Autodesk Inventor part; units mm, degrees
ref_plane "YZ Plane" through (0, 0, 0) normal (1, 0, 0) x (0, 1, 0)
ref_plane "XZ Plane" through (0, 0, 0) normal (0, 1, 0) x (-1, 0, 0)
ref_plane "XY Plane" through (0, 0, 0) normal (0, 0, 1) x (1, 0, 0)
sketch "Sketch1" plane through (0, 0, 0) normal (0, 1, 0) x (-1, 0, 0)
  line L0 (0, 0) -> (355.6, 0)
  line L1 (355.6, 0) -> (355.6, -406.4)
  line L2 (355.6, -406.4) -> (0, -406.4)
  line L3 (0, -406.4) -> (0, 0)
  dimension "d0" = 355.6
  dimension "d1" = 406.4
extrude "Extrusion1" add sketch "Sketch1" along normal blind 152.4
sketch "Sketch2" plane through (0, 152.4, 0) normal (0, 1, 0) x (1, 0, 0)
  line L0 (-355.6, 0) -> (0, 0)
  line L1 (0, 0) -> (0, 406.4)
  line L2 (0, 406.4) -> (-355.6, 406.4)
  line L3 (-355.6, 406.4) -> (-355.6, 0)
  line L4 (-1.5875, 1.5875) -> (-354.0125, 1.5875)
  line L5 (-354.0125, 1.5875) -> (-354.0125, 404.8125)
  line L6 (-354.0125, 404.8125) -> (-1.5875, 404.8125)
  line L7 (-1.5875, 404.8125) -> (-1.5875, 1.5875)
  dimension "d4" = 1.5875
  dimension "d5" = 1.5875
  dimension "d6" = 1.5875
  dimension "d7" = 1.5875
extrude "Extrusion2" cut sketch "Sketch2" against normal blind 150.8125 contours L4 L5 L6 L7
sketch "Sketch6" plane through (0, 0, 0) normal (1, 0, 0) x (0, 0, -1)
  line L0 (406.4, 0) -> (406.4, 152.4)
  line L1 (406.4, 0) -> (0, 0)
  circle A0 centre (337.3628, 87.884) radius 12.7
  dimension "d39" = 25.4
  dimension "d40" = 69.0372
  dimension "d41" = 87.884
extrude "Extrusion4" cut sketch "Sketch6" against normal up to surface (1.5875 mm away)
sketch "Sketch7" plane through (0, 0, -406.4) normal (0, 0, -1) x (-1, 0, 0)
  circle A0 centre (286.5628, 82.804) radius 12.7
  line L0 (355.6, 0) -> (0, 0)
  line L1 (0, 0) -> (0, 152.4)
  circle A1 centre (199.136, 69.85) radius 12.7
  line L2 (1.5875, 152.4) -> (1.5875, 1.5875)
  line L3 (355.6, 0) -> (355.6, 152.4)
  point P0 (1.5875, 0)
  dimension "d23" = 82.804
  dimension "d25" = 25.4
  dimension "d28" = 25.4
  dimension "d128" = 199.136
  dimension "d129" = 69.0372
  dimension "d154" = 69.85
extrude "Extrusion5" cut sketch "Sketch7" against normal blind 25.4
sketch "Sketch9" plane through (-355.6, 0, 0) normal (0, 0, 1) x (1, 0, 0)
  line L0 (25.4, 31.75) -> (330.2, 31.75)
  line L1 (330.2, 31.75) -> (330.2, 120.65)
  line L2 (330.2, 120.65) -> (25.4, 120.65)
  line L3 (25.4, 120.65) -> (25.4, 31.75)
  line L4 (355.6, 0) -> (355.6, 152.4)
  line L5 (355.6, 0) -> (0, 0)
  line L6 (0, 0) -> (0, 152.4)
  dimension "d61" = 304.8
  dimension "d62" = 88.9
  dimension "d64" = 31.75
  dimension "d110" = 355.6
  dimension "d111" = 25.4
extrude "Extrusion6" cut sketch "Sketch9" against normal blind 25.4
sketch "Sketch12" plane through (0, 0, -406.4) normal (0, 0, -1) x (-1, 0, 0)
  line L0 (50.8, 50.8) -> (105.918, 50.8)
  line L1 (105.918, 50.8) -> (105.918, 86.36)
  line L2 (105.918, 86.36) -> (50.8, 86.36)
  line L3 (50.8, 86.36) -> (50.8, 50.8)
  line L4 (63.7794, 81.9658) -> (92.9132, 81.9658)
  line L5 (0, 0) -> (0, 152.4)
  line L6 (355.6, 0) -> (0, 0)
  dimension "d120" = 35.56
  dimension "d121" = 55.118
  dimension "d122" = 50.8
  dimension "d123" = 50.8
extrude "Extrusion8" cut sketch "Sketch12" against normal blind 25.4
sketch "Sketch13" plane through (-355.6, 0, -406.4) normal (-1, 0, 0) x (0, 0, 1)
  circle A0 centre (123.0122, 82.804) radius 12.7
  circle A1 centre (69.0372, 87.884) radius 12.7
  circle A2 centre (69.0372, 87.884) radius 12.7
  line L0 (0, 0) -> (406.4, 0)
  line L1 (0, 0) -> (0, 152.4)
  line L2 (406.4, 152.4) -> (0, 152.4)
  line L3 (406.4, 0) -> (406.4, 152.4)
  dimension "d132" = 25.4
  dimension "d133" = 87.884
  dimension "d134" = 82.804
  dimension "d135" = 123.0122
extrude "Extrusion9" cut sketch "Sketch13" against normal up to surface (1.5875 mm away) contours A0
sketch "Sketch14" plane through (-355.6, 0, 0) normal (0, 0, 1) x (1, 0, 0)
  circle A0 centre (342.9, 120.65) radius 2.0828
  circle A1 centre (342.9, 31.75) radius 2.0828
  circle A2 centre (12.7, 31.75) radius 2.0828
  circle A3 centre (12.7, 120.65) radius 2.0828
  point P0 (355.6, 0)
hole "Hole1" at (-12.7, 120.65, 0) at (-12.7, 31.75, 0) at (-342.9, 31.75, 0) at (-342.9, 120.65, 0) direction (0, 0, -1) diameter 4.1656 depth 6.35 tip angle 118
sketch "Sketch15" plane through (0, 0, -406.4) normal (0, 0, -1) x (-1, 0, 0)
  circle A0 centre (40.64, 41.91) radius 1.7526
  circle A1 centre (116.84, 92.71) radius 1.7526
  circle A2 centre (40.64, 92.71) radius 1.7526
  circle A3 centre (116.84, 41.91) radius 1.7526
  circle A4 centre (56.261, 55.372) radius 2.1463
  circle A5 centre (101.219, 79.248) radius 2.1463
  circle A6 centre (101.219, 55.372) radius 2.1463
  circle A7 centre (56.261, 79.248) radius 2.1463
  arc A8 (64.1858, 79.0702) -> (57.8358, 72.7202) centre (64.1858, 72.7202) ccw
  line L0 (64.1858, 79.0702) -> (93.3196, 79.0702)
  arc A9 (99.6696, 72.7202) -> (93.3196, 79.0702) centre (93.3196, 72.7202) ccw
  line L1 (99.6696, 72.7202) -> (99.6696, 61.5442)
  arc A10 (93.3196, 55.1942) -> (99.6696, 61.5442) centre (93.3196, 61.5442) ccw
  line L2 (93.3196, 55.1942) -> (64.1858, 55.1942)
  arc A11 (57.8358, 61.5442) -> (64.1858, 55.1942) centre (64.1858, 61.5442) ccw
  line L3 (57.8358, 61.5442) -> (57.8358, 72.7202)
  line L4 (123.19, 99.06) -> (34.29, 99.06)
  line L5 (34.29, 99.06) -> (34.29, 35.56)
  line L6 (34.29, 35.56) -> (123.19, 35.56)
  line L7 (123.19, 35.56) -> (123.19, 99.06)
  line L8 (74.4123, 41.91) -> (73.7537, 41.91)
  line L9 (73.7537, 41.91) -> (73.7537, 47.6322)
  line L10 (73.7537, 47.6322) -> (72.6267, 47.6322)
  line L11 (72.6267, 47.6322) -> (72.6267, 48.2806)
  line L12 (72.6267, 48.2806) -> (75.7245, 48.2806)
  line L13 (75.7245, 48.2806) -> (75.7245, 47.6322)
  line L14 (75.7245, 47.6322) -> (74.5718, 47.6322)
  line L15 (74.5718, 47.6322) -> (74.5718, 43.3766)
  line L16 (74.5718, 43.3766) -> (75.7245, 43.3766)
  line L17 (75.7245, 43.3766) -> (75.7245, 42.7951)
  spline S0 degree 2 poles (75.7245, 42.7951) (75.071, 42.7951) (74.4535, 42.4246) (74.4123, 41.91) knots 0 0 0 1 2 2 2
  line L18 (82.8979, 42.6047) -> (84.2409, 42.6047)
  line L19 (84.2409, 42.6047) -> (84.2409, 41.9306)
  line L20 (84.2409, 41.9306) -> (82.0539, 41.9306)
  line L21 (82.0539, 41.9306) -> (82.0539, 46.6288)
  spline S1 degree 2 poles (82.0539, 46.6288) (82.0539, 47.4624) (83.0728, 48.3681) (83.9322, 48.3681) knots 0 0 0 1 2 2 2
  spline S2 degree 2 poles (83.9322, 48.3681) (84.138, 48.3681) (84.8224, 48.296) (85.054, 48.2446) knots 0 0 0 1 2 2 2
  line L22 (85.054, 48.2446) -> (85.054, 47.4315)
  line L23 (85.054, 47.4315) -> (85.0077, 47.4315)
  spline S3 degree 2 poles (85.0077, 47.4315) (84.8327, 47.4933) (84.313, 47.6373) (84.0454, 47.6373) knots 0 0 0 1 2 2 2
  spline S4 degree 2 poles (84.0454, 47.6373) (83.6543, 47.6373) (83.186, 47.4572) (83.078, 47.2926) knots 0 0 0 1 2 2 2
  spline S5 degree 2 poles (83.078, 47.2926) (82.9596, 47.1228) (82.8979, 46.6288) (82.8979, 46.3046) knots 0 0 0 1 2 2 2
  line L24 (82.8979, 46.3046) -> (82.8979, 42.6047)
  spline S6 degree 2 poles (80.4896, 42.7951) (79.8361, 42.7951) (79.2186, 42.4246) (79.1774, 41.91) knots 0 0 0 1 2 2 2
  line L25 (79.1774, 41.91) -> (78.5187, 41.91)
  line L26 (78.5187, 41.91) -> (78.5187, 47.6322)
  line L27 (78.5187, 47.6322) -> (77.3918, 47.6322)
  line L28 (77.3918, 47.6322) -> (77.3918, 48.2806)
  line L29 (77.3918, 48.2806) -> (80.4896, 48.2806)
  line L30 (80.4896, 48.2806) -> (80.4896, 47.6322)
  line L31 (80.4896, 47.6322) -> (79.3369, 47.6322)
  line L32 (79.3369, 47.6322) -> (79.3369, 43.3766)
  line L33 (79.3369, 43.3766) -> (80.4896, 43.3766)
  line L34 (80.4896, 43.3766) -> (80.4896, 42.7951)
  point P0 (0, 0)
hole "Hole2" at (-116.84, 92.71, -406.4) at (-116.84, 41.91, -406.4) at (-40.64, 41.91, -406.4) at (-40.64, 92.71, -406.4) direction (0, 0, 1) diameter 4.1656 depth 6.35 tip angle 118
thread "Thread1"
thread "Thread2"
thread "Thread3"
thread "Thread4"
thread "Thread5"
thread "Thread6"
thread "Thread7"
thread "Thread8"
equation "\"d5\" = d4"
equation "\"d6\" = d4"
equation "\"d7\" = d4"
equation "\"d28\" = d25"
equation "\"d26\" = d28"
equation "\"d111\" = -0.5 * d61 + 0.5 * d110"
properties part number "18x12x6Box"
For this review, take the finished solid that the model builds, in its own axes (mm). A direction names the side the tool comes from. Give positions to 0.01 mm unless a question says otherwise; leave off trailing zeros. Order: outer loops, then holes, each group sorted by start corner. A loop starts at its lowest first (then second) coordinate and runs counter-clockwise, first axis right, second up. Notation, with made-up numbers: (63.5, 8.25) - (72.5, 8.25) arc R18 ccw to (72.5, 28.25) - close; hole circle Ø6 at (20, -15.75). An arc over 180 degrees is marked (long way). Answer as a JSON object with one key per item and string values. Group by question number.
Item 1: Wall thickness on line 1 along Y through (x, z) = (-40.64, -405.5); line 2 along Y through (x, z) = (-342.9, -1.2); line 3 along Z through (x, y) = (-336, 95.5): over which ranges is each line inside the solid? List them lowest first.
Item 2: Take a section at A-A on y = 20.5. Give the boundary of the cut face in (x, z).
Item 3: Take a section at C-C on z = -264.5. Give the boundary of the cut face in (x, y).
Item 4: Clearance check with flat-ended pins moving along their axes: pin 1 Ø15 at (y, z) = (82.8, -283.39) entering from -X; pin 2 Ø20.5 at (x, y) = (-199.136, 69.85) entering from -Z; pin 3 Ø10 at (x, z) = (-153, -59.5) entering from +Y; pin 4 Ø5.5 at (x, y) = (-116.84, 41.91) entering from +Z. State where each tip first meets the part, or that it passes through.
Item 5: Draft analysis for pull direction X (two halves, no side actions). For faces 4 (the cylindrical face through (-354.817, 83.362, -296.076)), 5 (the flat face through (-355.6, 75, -200)), 6 (the cylindrical face through (-298.676, 86.619, -405.617)), state which applies: pulls with the +X half, pulls with the -X half, needs draft (parallel to the pull), parting line crosses it, or undercut.
Item 6: Machinability: for faces 1 (the flat face through (-175, 0, -200)), 2 (the flat face through (-1.588, 78, -206)), 3 (the cylindrical face through (-0.783, 88.442, -324.675)), which of the approach directions +Z, -Z, +X, -X, +Y, -Y give a long, thin tool a straight path to every point of the face, cutting with its end or side? Answer none if there is none.
Item 7: Take a section at B-B on x = -157.5. Give the boundary of the cut face in (y, z).
Reported:
{
 "1": {"line 1": "0 to 39.83, 43.99 to 90.63, 94.79 to 152.4", "line 2": "0 to 29.67, 33.83 to 118.57, 122.73 to 152.4", "line 3": "-406.4 to -404.81, -1.59 to 0"},
 "2": {"outline": "(-355.6, -406.4) - (0, -406.4) - (0, 0) - (-355.6, 0) - close; hole (-354.01, -404.81) - (-1.59, -404.81) - (-1.59, -1.59) - (-354.01, -1.59) - close"},
 "3": {"outline": "(-355.6, 0) - (0, 0) - (0, 152.4) - (-1.59, 152.4) - (-1.59, 1.59) - (-354.01, 1.59) - (-354.01, 152.4) - (-355.6, 152.4) - close"},
 "4": {"pin 1": "x = -1.59", "pin 2": "through", "pin 3": "y = 1.59", "pin 4": "z = -404.81"},
 "5": {"face 4": "needs draft", "face 5": "pulls with the -X half", "face 6": "undercut"},
 "6": {"face 1": "+Z, -Z, +X, -X, -Y", "face 2": "+Y", "face 3": "+X"},
 "7": {"outline": "(0, -406.4) - (152.4, -406.4) - (152.4, -404.81) - (1.59, -404.81) - (1.59, -1.59) - (31.75, -1.59) - (31.75, 0) - (0, 0) - close; (120.65, -1.59) - (152.4, -1.59) - (152.4, 0) - (120.65, 0) - close"}
}
